Here's how the part is built. I have some questions about the finished solid (model axes, mm). Round coordinates to 2 decimals unless told otherwise and drop trailing zeros. Loops run counter-clockwise (first coordinate to the right, second up) from the corner with the lowest first, then second, coordinate; pieces in that order, holes last. Notation, with made-up numbers: M 83,16.25 L 116,16.25 A19 cw 116,36.25 Z; hole C 12.25,42.25 d2. An arc over 180 degrees is marked long. Answer as CSV lines item,"result".
```python
from build123d import *

# Parameters (mm, degrees)
PLATE_OUTLITE_BOSS_EXTRUDE_DEPTH                  = 9.53
BEAM_CLEARANCE_HOLE_REACH                         = 11.53
SKETCH2_R                                         = 135
A_6_2_6_2_DIAMETER_HOLE_D                         = 6.2
A_6_2_6_2_DIAMETER_HOLE_DEPTH                     = 9.53
B_TAP_DRILL_FOR_M6X1_0_TAP_D                      = 5
B_TAP_DRILL_FOR_M6X1_0_TAP_DEPTH                  = 9.53
C_12_5_12_5_DIAMETER_HOLE_D                       = 12.7
C_12_5_12_5_DIAMETER_HOLE_DEPTH                   = 9.53
E_6_2_6_2_DIAMETER_HOLE_D                         = 6.2
E_6_2_6_2_DIAMETER_HOLE_DEPTH                     = 9.53
F_TAP_DRILL_FOR_M8X1_25_TAP_D                     = 6.8
F_TAP_DRILL_FOR_M8X1_25_TAP_DEPTH                 = 9.53
J_6_0_6_DIAMETER_HOLE_D                           = 6
J_6_0_6_DIAMETER_HOLE_DEPTH                       = 9.53
K_10_0_10_DIAMETER_HOLE_D                         = 10
K_10_0_10_DIAMETER_HOLE_DEPTH                     = 9.53
L_6_1MM_HOLE_9_53MM_C_BORE_3_2MM_DEEP_D           = 6.1
L_6_1MM_HOLE_9_53MM_C_BORE_3_2MM_DEEP_DEPTH       = 9.53
L_6_1MM_HOLE_9_53MM_C_BORE_3_2MM_DEEP_CBORE_D     = 9.53
L_6_1MM_HOLE_9_53MM_C_BORE_3_2MM_DEEP_CBORE_DEPTH = 3.2
L_6_1MM_HOLE_9_53MM_C_BORE_3_2MM_DEEP_TIP         = 1.832624888
M_6_0_6_DIAMETER_HOLE_D                           = 6
M_6_0_6_DIAMETER_HOLE_DEPTH                       = 10
M_6_0_6_DIAMETER_HOLE_TIP                         = 1.802581857


with BuildPart() as part:
    # Sketch1 → Plate Outlite - Boss-Extrude (new body)
    with BuildSketch(Plane(origin=(0, 0, 0), x_dir=(1, 0, 0), z_dir=(0, 1, 0))):
        Polygon((-260, 240), (226, 240), (816, 515.1), (1080.6, 515.1), (1080.6, 355.1), (971, 355.1), (136, -570), (-260, -570), align=None)
    extrude(amount=PLATE_OUTLITE_BOSS_EXTRUDE_DEPTH)

    # Sketch2 → Beam Clearance Hole (cut, up to next)
    with BuildSketch(Plane(origin=(0, 9.53, 0), x_dir=(1, 0, 0), z_dir=(0, 1, 0)), mode=Mode.PRIVATE) as beam_clearance_hole_sk1:
        Circle(SKETCH2_R)
    beam_clearance_hole_tool1 = extrude(beam_clearance_hole_sk1.sketch, amount=-BEAM_CLEARANCE_HOLE_REACH, mode=Mode.PRIVATE) & part.part
    add(beam_clearance_hole_tool1.solids().sort_by_distance((0, 9.53, 0))[0], mode=Mode.SUBTRACT)

    # A - Ø6.2 (6.2) Diameter Hole
    with Locations(Plane(origin=(0, 9.53, 0), x_dir=(1, 0, 0), z_dir=(0, 1, 0))):
        with Locations((-190, 190), (190, 190), (190, -190), (-190, -190), (-190, -500), (190, -500)):
            Hole(A_6_2_6_2_DIAMETER_HOLE_D / 2, depth=A_6_2_6_2_DIAMETER_HOLE_DEPTH)

    # B - Tap Drill for M6x1.0 Tap
    with Locations(Plane(origin=(0, 9.53, 0), x_dir=(1, 0, 0), z_dir=(0, 1, 0))):
        with Locations((-80, 220), (80, 220), (524.5, 212.5), (979.9, 495.2), (1043.4, 465.7), (971, 398.8), (761.6, 412), (826.04, 335.57), (684.8, 177.3), (601, 276.7), (608.3, 112.8), (80, -555), (-80, -555), (740.8, 172.5), (631.6, 302.5)):
            Hole(B_TAP_DRILL_FOR_M6X1_0_TAP_D / 2, depth=B_TAP_DRILL_FOR_M6X1_0_TAP_DEPTH)

    # C - Ø12.5 (12.5) Diameter Hole
    with Locations(Plane(origin=(0, 9.53, 0), x_dir=(1, 0, 0), z_dir=(0, 1, 0))):
        with Locations((-245, 210), (-245, -210), (245, -210), (245, 210)):
            Hole(C_12_5_12_5_DIAMETER_HOLE_D / 2, depth=C_12_5_12_5_DIAMETER_HOLE_DEPTH)

    # E - Ø6.2 (6.2) Diameter Hole
    with Locations(Plane(origin=(0, 9.53, 0), x_dir=(1, 0, 0), z_dir=(0, 1, 0))):
        with Locations((935.6, 500.1), (1045.6, 500.1), (1045.6, 370.1), (935.6, 370.1)):
            Hole(E_6_2_6_2_DIAMETER_HOLE_D / 2, depth=E_6_2_6_2_DIAMETER_HOLE_DEPTH)

    # F - Tap Drill for M8x1.25 Tap
    with Locations(Plane(origin=(0, 9.53, 0), x_dir=(1, 0, 0), z_dir=(0, 1, 0))):
        with Locations((-120, 145), (120, 145), (0, -160), (-134.9, -298.7), (-179.1, -393.9), (120.1, -533), (164.4, -437.8)):
            Hole(F_TAP_DRILL_FOR_M8X1_25_TAP_D / 2, depth=F_TAP_DRILL_FOR_M8X1_25_TAP_DEPTH)

    # J - Ø6.0 (6) Diameter Hole
    with Locations(Plane(origin=(0, 9.53, 0), x_dir=(1, 0, 0), z_dir=(0, 1, 0))):
        with Locations((200, 225.1), (474.5, 0), (738.3, 222.4), (590.6, 225.1)):
            Hole(J_6_0_6_DIAMETER_HOLE_D / 2, depth=J_6_0_6_DIAMETER_HOLE_DEPTH)

    # K - Ø10.0 (10) Diameter Hole
    with Locations(Plane(origin=(0, 9.53, 0), x_dir=(1, 0, 0), z_dir=(0, 1, 0))):
        with Locations((0, -190), (0, -400)):
            Hole(K_10_0_10_DIAMETER_HOLE_D / 2, depth=K_10_0_10_DIAMETER_HOLE_DEPTH)

    # L - 6.1mm Hole, 9.53mm C-bore 3.2mm deep
    with Locations(Plane(origin=(0, 9.53, 0), x_dir=(1, 0, 0), z_dir=(0, 1, 0))):
        with Locations((740.6, 435.1)):
            CounterBoreHole(L_6_1MM_HOLE_9_53MM_C_BORE_3_2MM_DEEP_D / 2, L_6_1MM_HOLE_9_53MM_C_BORE_3_2MM_DEEP_CBORE_D / 2, L_6_1MM_HOLE_9_53MM_C_BORE_3_2MM_DEEP_CBORE_DEPTH, depth=L_6_1MM_HOLE_9_53MM_C_BORE_3_2MM_DEEP_DEPTH)
            with Locations((0, 0, -(L_6_1MM_HOLE_9_53MM_C_BORE_3_2MM_DEEP_DEPTH + L_6_1MM_HOLE_9_53MM_C_BORE_3_2MM_DEEP_TIP / 2))):  # 118° drill point
                Cone(0, L_6_1MM_HOLE_9_53MM_C_BORE_3_2MM_DEEP_D / 2, L_6_1MM_HOLE_9_53MM_C_BORE_3_2MM_DEEP_TIP, mode=Mode.SUBTRACT)

    # M - Ø6.0 (6) Diameter Hole
    with Locations(Plane(origin=(0, 9.53, 0), x_dir=(1, 0, 0), z_dir=(0, 1, 0))):
        with Locations((990.6, 435.1)):
            Hole(M_6_0_6_DIAMETER_HOLE_D / 2, depth=M_6_0_6_DIAMETER_HOLE_DEPTH)
            with Locations((0, 0, -(M_6_0_6_DIAMETER_HOLE_DEPTH + M_6_0_6_DIAMETER_HOLE_TIP / 2))):  # 118° drill point
                Cone(0, M_6_0_6_DIAMETER_HOLE_D / 2, M_6_0_6_DIAMETER_HOLE_TIP, mode=Mode.SUBTRACT)


solid = part.part
```
1. For P1, Ø5, axis at y = 4, z = -159.5, coming from the +X side; P2, Ø7, axis at x = 1045.6, z = -370.1, coming from the +Y side; P3, Ø1.5, axis at y = 7.5, z = -92, coming from the +X side, each with a flat end and sliding along its axis, tell me the tip position at first contact or that it passes through.
Evaluation:
P1,"stops at x = 796.71"
P2,"stops at y = 9.53"
P3,"stops at x = 734.2"
2. I want a section at B-B, the plane x = 337. Please give me the cut outline in (y, z), and give its area (3 significant figures).
Evaluation:
outline,"M 0,-291.76 L 9.53,-291.76 L 9.53,347.31 L 0,347.31 Z"
area,"6,090 mm²"
3. If I drill on line 1 (X direction, y = 8.5, z = -370); line 2 (X direction, y = 0.5, z = 209.5); line 3 (Z direction, x = 1045.6, y = 5.25), over which ranges is the centre line in solid material (lowest first)? Write a range as [from, to].
Evaluation:
line 1,"x = [504.81, 932.5], [938.7, 1042.5], [1048.7, 1080.6]"
line 2,"x = [-260, -251.33], [-238.67, 238.67], [251.33, 461.39]"
line 3,"z = [-515.1, -503.2], [-497, -466.89], [-464.51, -373.2], [-367, -355.1]"
4. I want a section at A-A, the plane y = 3.5. Count the separate pieces of the cut face and the enclosed holes in it, and give its area (3 significant figures).
Evaluation:
separate pieces,"1"
enclosed holes,"45"
area,"693,000 mm²"
